from build123d import *

# Parameters (mm, degrees)
CROQUIS2_W               = 240
CROQUIS2_H               = 240
CROQUIS2_W_2             = 232
CROQUIS2_H_2             = 232
SALIENTE_EXTRUIR1_DEPTH  = 45
CROQUIS4_W               = 8.5
CROQUIS4_H               = 10
SALIENTE_EXTRUIR2_DEPTH  = 15
CORTAR_EXTRUIR1_REACH    = 187.373
CROQUIS5_R               = 1
CORTAR_EXTRUIR2_REACH    = 187.876
CROQUIS6_W               = 3.5
CROQUIS6_H               = 10
SALIENTE_EXTRUIR3_DEPTH  = 240
CORTAR_EXTRUIR3_DEPTH    = 250
SALIENTE_EXTRUIR4_DEPTH  = 240
CORTAR_EXTRUIR4_DEPTH    = 250
CROQUIS11_W              = 54
CROQUIS11_H              = 54
CROQUIS11_W_2            = 50
CROQUIS11_H_2            = 50
SALIENTE_EXTRUIR5_DEPTH  = 30
CORTAR_EXTRUIR5_START    = -54
CORTAR_EXTRUIR5_DEPTH    = 54
CROQUIS14_W              = 240
CROQUIS14_H              = 45
SALIENTE_EXTRUIR6_DEPTH  = 5
CROQUIS15_W              = 245
CROQUIS15_H              = 45
SALIENTE_EXTRUIR7_DEPTH  = 5
CROQUIS16_W              = 245
CROQUIS16_H              = 45
SALIENTE_EXTRUIR8_DEPTH  = 5
CROQUIS17_W              = 250
CROQUIS17_H              = 45
SALIENTE_EXTRUIR9_DEPTH  = 5
CROQUIS18_W              = 242
CROQUIS18_H              = 242
CORTAR_EXTRUIR6_DEPTH    = 43
SALIENTE_EXTRUIR10_DEPTH = 28
CORTAR_EXTRUIR7_REACH    = 213.906
CROQUIS20_R              = 3.9


# Read off the part's stored shape, not the designer's step: Cortar-Extruir5
with BuildPart() as part:
    # Croquis2 → Saliente-Extruir1 (new body)
    with BuildSketch(Plane(origin=(0, 0, 0), x_dir=(1, 0, 0), z_dir=(0, 1, 0))):
        with Locations((5, 5)):
            Rectangle(CROQUIS2_W, CROQUIS2_H)
        with Locations((5, 5)):
            Rectangle(CROQUIS2_W_2, CROQUIS2_H_2, mode=Mode.SUBTRACT)
    extrude(amount=SALIENTE_EXTRUIR1_DEPTH)

    # Croquis4 → Saliente-Extruir2 (add)
    with BuildSketch(Plane.XY.offset(115)):
        with Locations((5, 25)):
            Rectangle(CROQUIS4_W, CROQUIS4_H)
    extrude(amount=SALIENTE_EXTRUIR2_DEPTH)

    # Croquis5 → Cortar-Extruir1 (cut, up to next)
    with BuildSketch(Plane(origin=(9.25, 0, 0), x_dir=(0, 0, -1), z_dir=(1, 0, 0)), mode=Mode.PRIVATE) as cortar_extruir1_sk1:
        with Locations(Location((-126, 26, 0), (0, 0, 90))):
            Circle(CROQUIS5_R)
    cortar_extruir1_tool1 = extrude(cortar_extruir1_sk1.sketch, amount=-CORTAR_EXTRUIR1_REACH, mode=Mode.PRIVATE) & part.part
    add(cortar_extruir1_tool1.solids().sort_by_distance((9.25, 26, 126))[0], mode=Mode.SUBTRACT)

    # Croquis6 → Cortar-Extruir2 (cut, up to next)
    with BuildSketch(Plane(origin=(0, 45, 0), x_dir=(1, 0, 0), z_dir=(0, 1, 0)), mode=Mode.PRIVATE) as cortar_extruir2_sk1:
        with Locations((5, -125)):
            Rectangle(CROQUIS6_W, CROQUIS6_H)
    cortar_extruir2_tool1 = extrude(cortar_extruir2_sk1.sketch, amount=-CORTAR_EXTRUIR2_REACH, mode=Mode.PRIVATE) & part.part
    add(cortar_extruir2_tool1.solids().sort_by_distance((5, 45, 125))[0], mode=Mode.SUBTRACT)

    # Croquis7 → Saliente-Extruir3 (add)
    with BuildSketch(Plane.ZY.offset(115)):
        Polygon((113, 0), (115, 0), (22, -40), (20, -40), align=None)
        Polygon((-125, 0), (-123, 0), (-30, -40), (-32, -40), align=None)
    extrude(amount=-SALIENTE_EXTRUIR3_DEPTH)

    # Croquis8 → Cortar-Extruir3 (cut)
    with BuildSketch(Plane.XY.offset(115)):
        Polygon((123, 0), (30, -40), (125, -40), (125, 0), align=None)
        Polygon((-115, -40), (-20, -40), (-113, 0), (-115, 0), align=None)
    extrude(amount=-CORTAR_EXTRUIR3_DEPTH, mode=Mode.SUBTRACT)

    # Croquis9 → Saliente-Extruir4 (add)
    with BuildSketch(Plane(origin=(0, 0, -125), x_dir=(-1, 0, 0), z_dir=(0, 0, -1))):
        Polygon((20, -40), (22, -40), (115, 0), (113, 0), align=None)
        Polygon((-30, -40), (-32, -40), (-125, 0), (-123, 0), align=None)
    extrude(amount=-SALIENTE_EXTRUIR4_DEPTH)

    # Croquis10 → Cortar-Extruir4 (cut)
    with BuildSketch(Plane.ZY.offset(115)):
        Polygon((-125, -40), (-125, 0), (-32, -40), align=None)
        Polygon((22, -40), (115, -40), (115, 0), align=None)
    extrude(amount=-CORTAR_EXTRUIR4_DEPTH, mode=Mode.SUBTRACT)

    # Croquis11 → Saliente-Extruir5 (add)
    with BuildSketch(Plane.XZ.offset(40)):
        with Locations((5, -5)):
            Rectangle(CROQUIS11_W, CROQUIS11_H)
        with Locations((5, -5)):
            Rectangle(CROQUIS11_W_2, CROQUIS11_H_2, mode=Mode.SUBTRACT)
    extrude(amount=SALIENTE_EXTRUIR5_DEPTH)

    # Cortar-Extruir5 outline → Cortar-Extruir5 (cut)
    with BuildSketch(Plane(origin=(32, 0, 0), x_dir=(0, 0, -1), z_dir=(1, 0, 0)).offset(CORTAR_EXTRUIR5_START)):
        Polygon((-22, -70), (32, -70), (-22, -69.999), align=None)
    extrude(amount=CORTAR_EXTRUIR5_DEPTH, mode=Mode.SUBTRACT)

    # Croquis14 → Saliente-Extruir6 (add)
    with BuildSketch(Plane.XY.offset(115)):
        with Locations((5, 22.5)):
            Rectangle(CROQUIS14_W, CROQUIS14_H)
    extrude(amount=SALIENTE_EXTRUIR6_DEPTH)

    # Croquis15 → Saliente-Extruir7 (add)
    with BuildSketch(Plane(origin=(125, 0, 0), x_dir=(0, 0, -1), z_dir=(1, 0, 0))):
        with Locations((2.5, 22.5)):
            Rectangle(CROQUIS15_W, CROQUIS15_H)
    extrude(amount=SALIENTE_EXTRUIR7_DEPTH)

    # Croquis16 → Saliente-Extruir8 (add)
    with BuildSketch(Plane(origin=(0, 0, -125), x_dir=(-1, 0, 0), z_dir=(0, 0, -1))):
        with Locations((-7.5, 22.5)):
            Rectangle(CROQUIS16_W, CROQUIS16_H)
    extrude(amount=SALIENTE_EXTRUIR8_DEPTH)

    # Croquis17 → Saliente-Extruir9 (add)
    with BuildSketch(Plane.ZY.offset(115)):
        with Locations((-5, 22.5)):
            Rectangle(CROQUIS17_W, CROQUIS17_H)
    extrude(amount=SALIENTE_EXTRUIR9_DEPTH)

    # Croquis18 → Cortar-Extruir6 (cut)
    with BuildSketch(Plane(origin=(0, 45, 0), x_dir=(1, 0, 0), z_dir=(0, 1, 0))):
        with Locations((5, 5)):
            Rectangle(CROQUIS18_W, CROQUIS18_H)
    extrude(amount=-CORTAR_EXTRUIR6_DEPTH, mode=Mode.SUBTRACT)

    # Croquis19 → Saliente-Extruir10 (add)
    with BuildSketch(Plane(origin=(32, 0, 0), x_dir=(0, 0, -1), z_dir=(1, 0, 0))):
        Polygon((32, -70), (32, -68), (-9.324230876, -68), (-9.324230876, -69.999234736), align=None)
    extrude(amount=SALIENTE_EXTRUIR10_DEPTH)

    # Croquis20 → Cortar-Extruir7 (cut, up to next)
    with BuildSketch(Plane(origin=(32, 0, 0), x_dir=(0, 0, -1), z_dir=(1, 0, 0)), mode=Mode.PRIVATE) as cortar_extruir7_sk1:
        with Locations((26.058589575, -62)):
            Circle(CROQUIS20_R)
    cortar_extruir7_tool1 = extrude(cortar_extruir7_sk1.sketch, amount=-CORTAR_EXTRUIR7_REACH, mode=Mode.PRIVATE) & part.part
    add(cortar_extruir7_tool1.solids().sort_by_distance((32, -62, -26.05859))[0], mode=Mode.SUBTRACT)


solid = part.part
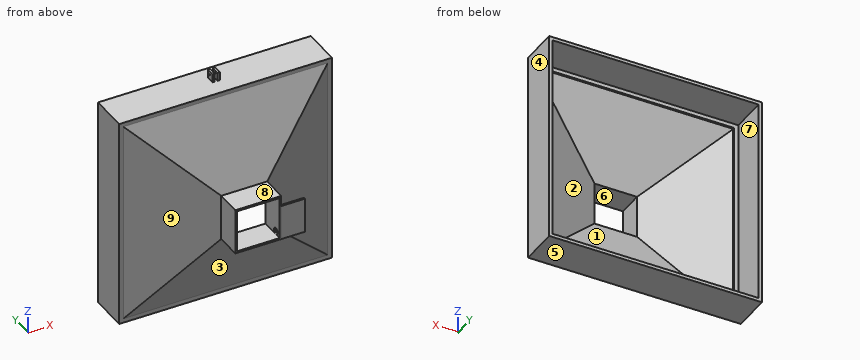
Can you work these out from the model? Positions are in its coordinate system, mm. Face numbers are marked on the shaded views. A direction names the side the tool comes from. Give positions to 0.01 mm unless a question says otherwise; leave off trailing zeros. Order: outer loops, then holes, each group sorted by start corner. A loop starts at its lowest first (then second) coordinate and runs counter-clockwise, first axis right, second up. Notation, with made-up numbers: M -18.5,31 L -2.5,31 A27 cw -2.5,67 Z; hole C 60.25,-26.5 d8. An arc over 180 degrees is marked long. Use a Markdown table: item, result. Add a question column.
Item 1: For the marked faces 5, 6, 7, 8 and 9, which set-ups out of +Z, -Z, +X, -X, +Y, -Y let a thin tool reach every point of the face, with its end or its side?
Item 2: If I drill on L1, parallel to Z at x = 7.4, y = 26; L2, parallel to X at y = 20.5, z = -3; L3, parallel to Z at x = -14, y = 4.5, over which ranges is the centre line in solid material (lowest first)? Write a range as [from, to].
Item 3: Will these pins go through, and if not, where does the flat tip stop? pin 1 (1.6 mm diameter, centred on y = -69, z = -2.5, fed in from +X); pin 2 (24 mm diameter, centred on x = 0, y = -62, fed in from +Z); pin 3 (10 mm diameter, centred on x = -92, y = -17, fed in from -Z); pin 4 (24 mm diameter, centred on y = -59, z = -6, fed in from -X).
Item 4: Suppose I cut it at B-B (z = -6). List the corners of the cut face in (x, y) for me, then the cut area to 3 significant figures.
Item 5: Suppose I cut it at D-D (x = -33). List the corners of the cut face in (y, z) for me.
Item 6: We'd pull the mould along Z, two halves only. Please class the marked faces 1, 2, 3 and 4: +Z half, -Z half, draft (parallel to the pull), parting line (faces both ways), or undercut.
Item 7: Suppose I cut it at A-A (y = -62). List the corners of the cut face in (x, z) for me.
Item 8: Suppose I cut it at C-C (y = -44.5). List the corners of the cut face in (x, z) for me, then the cut area to 3 significant figures.
Answer sheet:
| question | item | result |
|---|---|---|
| 1 | face 5 | -Z, +X, -X, +Y, -Y |
| 1 | face 6 | +Y, -Y |
| 1 | face 7 | +Y |
| 1 | face 8 | +Z, +X, -X, -Y |
| 1 | face 9 | +Z, -Z, -X, -Y |
| 2 | L1 | z = [-130, -126], [116, 125], [127, 130] |
| 2 | L2 | x = [-120, -116], [126, 130] |
| 2 | L3 | z = [-130, -126], [116, 120] |
| 3 | pin 1 | stops at x = 60 |
| 3 | pin 2 | stops at z = 22 |
| 3 | pin 3 | passes through |
| 3 | pin 4 | stops at x = -22 |
| 4 | outline | M -120,0 L -115,0 L -22,-40 L -22,-70 L -20,-70 L -20,-40 L -113,0 L -111,0 L -111,2 L -116,2 L -116,45 L -120,45 Z; M 30,-70 L 60,-70 L 60,-68 L 32,-68 L 32,-40 L 125,0 L 130,0 L 130,45 L 126,45 L 126,2 L 121,2 L 121,0 L 123,0 L 30,-40 Z |
| 4 | area | 716 mm² |
| 5 | outline | M -35.27,-43 L 0,-125 L 0,-130 L 45,-130 L 45,-126 L 2,-126 L 2,-121 L 0,-121 L 0,-123 L -34.41,-43 L -34.41,33 L 0,113 L 0,111 L 2,111 L 2,116 L 45,116 L 45,120 L 0,120 L 0,115 L -35.27,33 Z |
| 6 | face 1 | undercut |
| 6 | face 2 | undercut |
| 6 | face 3 | -Z half |
| 6 | face 4 | draft |
| 7 | outline | M -22,-32 L 32,-32 L 32,-29.96 L 30,-29.96 L 30,-30 L -20,-30 L -20,20 L 30,20 L 30,-22.16 L 32,-22.16 L 32,22 L -22,22 Z |
| 8 | outline | M -22,-32 L 32,-32 L 32,22 L -22,22 Z; hole M -20,-30 L 30,-30 L 30,20 L -20,20 Z |
| 8 | area | 416 mm² |
